```python
from build123d import *

# Parameters (mm, degrees)
SKETCH1_W                                    = 152.4
SKETCH1_H                                    = 88.9
BASE_FLANGE1_DEPTH                           = 1.29032
EDGE_FLANGE1_STRIP_W                         = 5.85978
EDGE_FLANGE1_STRIP_H                         = 1.29032
EDGE_FLANGE1_STRIP_CUT_DEPTH                 = 88.9
EDGE_FLANGE1_STRIP_2_W                       = 5.85978
EDGE_FLANGE1_STRIP_2_H                       = 1.29032
EDGE_FLANGE1_STRIP_CUT_2_DEPTH               = 88.9
EDGE_FLANGE1_DEPTH                           = 88.9
EDGE_FLANGE1_BEND_DEPTH                      = 88.9
F_4_22MM_HOLE_FOR_M3_CLINCH_NUT_D            = 4.22
BREAK_CORNER1_START                          = -77.68082
BREAK_CORNER1_DEPTH                          = 155.36164
CUT_THICKEN1_START                           = 41.91
CUT_THICKEN1_OUTLINE_W                       = 0.127
CUT_THICKEN1_OUTLINE_H                       = 1.29032
CUT_THICKEN1_DEPTH                           = 2.54
CUT_THICKEN2_START                           = 41.91
CUT_THICKEN2_OUTLINE_W                       = 0.127
CUT_THICKEN2_OUTLINE_H                       = 1.29032
CUT_THICKEN2_DEPTH                           = 2.54
MIRROR7_START                                = 41.91
MIRROR7_COPY_1_SKETCH_W                      = 0.127
MIRROR7_COPY_1_SKETCH_H                      = 1.29032
MIRROR7_COPY_1_DEPTH                         = 2.54
MIRROR7_COPY_2_SKETCH_W                      = 0.127
MIRROR7_COPY_2_SKETCH_H                      = 1.29032
MIRROR7_COPY_2_DEPTH                         = 2.54
MOVE_FACE1_BY                                = 1.27
MOVE_FACE1_2_BY                              = 1.27
MOVE_FACE1_3_BY                              = 1.27
MOVE_FACE1_4_BY                              = 1.27
EDGE_FLANGE2_STRIP_W                         = 5.66928
EDGE_FLANGE2_STRIP_H                         = 1.29032
EDGE_FLANGE2_STRIP_CUT_DEPTH                 = 2.54
EDGE_FLANGE2_STRIP_2_W                       = 5.66928
EDGE_FLANGE2_STRIP_2_H                       = 1.29032
EDGE_FLANGE2_STRIP_CUT_2_DEPTH               = 2.54
EDGE_FLANGE2_STRIP_3_W                       = 5.66928
EDGE_FLANGE2_STRIP_3_H                       = 1.29032
EDGE_FLANGE2_STRIP_CUT_3_DEPTH               = 2.54
EDGE_FLANGE2_STRIP_4_W                       = 5.66928
EDGE_FLANGE2_STRIP_4_H                       = 1.29032
EDGE_FLANGE2_STRIP_CUT_4_DEPTH               = 2.54
EDGE_FLANGE2_DEPTH                           = 2.54
EDGE_FLANGE2_BEND_DEPTH                      = 2.54
EDGE_FLANGE2_BEND_2_DEPTH                    = 2.54
EDGE_FLANGE2_BEND_3_DEPTH                    = 2.54
CHANGE_START                                 = -77.68082
CHANGE_NOTE_FOR_REVH_TO_ADD_010_CLEARA_DEPTH = 155.36164


# Read off the part's stored shape, not the designer's step: Break-Corner1, Cut-Thicken1, Cut-Thicken2, change note for revH to add .010" clearance
# Sheet-metal steps are written as plain solids
with BuildPart() as part:
    # Sketch1 → Base-Flange1 (new body)
    with BuildSketch(Plane.XY):
        Rectangle(SKETCH1_W, SKETCH1_H)
    extrude(amount=-BASE_FLANGE1_DEPTH)

    # Edge-Flange1 strip (across the edge) → Edge-Flange1 strip cut (cut)
    with BuildSketch(Plane(origin=(-76.3905, -44.45, -1.29032), x_dir=(1, 0, 0), z_dir=(0, 1, 0))):
        with Locations((-2.67589, -0.64516)):
            Rectangle(EDGE_FLANGE1_STRIP_W, EDGE_FLANGE1_STRIP_H)
    extrude(amount=EDGE_FLANGE1_STRIP_CUT_DEPTH, mode=Mode.SUBTRACT)

    # Edge-Flange1 strip 2 (across the edge) → Edge-Flange1 strip cut 2 (cut)
    with BuildSketch(Plane(origin=(76.3905, 44.45, -1.29032), x_dir=(-1, 0, 0), z_dir=(0, -1, 0))):
        with Locations((-2.67589, -0.64516)):
            Rectangle(EDGE_FLANGE1_STRIP_2_W, EDGE_FLANGE1_STRIP_2_H)
    extrude(amount=EDGE_FLANGE1_STRIP_CUT_2_DEPTH, mode=Mode.SUBTRACT)

    # Edge-Flange1 section (across the edge) → Edge-Flange1 (add)
    with BuildSketch(Plane(origin=(-76.3905, -44.45, -1.29032), x_dir=(1, 0, 0), z_dir=(0, 1, 0))):
        with BuildLine():
            Line((-1.29032, 0.254), (-1.29032, 46.96968))
            Line((-1.29032, 46.96968), (0, 46.96968))
            Line((0, 46.96968), (0, 0.254))
            ThreePointArc((0, 0.254), (0.074394878, 0.074394878), (0.254, 0))
            Line((0.254, 0), (0.254, -1.29032))
            ThreePointArc((0.254, -1.29032), (-0.837999144, -0.837999144), (-1.29032, 0.254))
        make_face()
    extrude(amount=EDGE_FLANGE1_DEPTH)

    # Edge-Flange1 section 2 (across the edge) → Edge-Flange1 bend (add)
    with BuildSketch(Plane(origin=(76.3905, 44.45, -1.29032), x_dir=(-1, 0, 0), z_dir=(0, -1, 0))):
        with BuildLine():
            Line((-1.29032, 0.254), (-1.29032, 46.96968))
            Line((-1.29032, 46.96968), (0, 46.96968))
            Line((0, 46.96968), (0, 0.254))
            ThreePointArc((0, 0.254), (0.074394878, 0.074394878), (0.254, 0))
            Line((0.254, 0), (0.254, -1.29032))
            ThreePointArc((0.254, -1.29032), (-0.837999144, -0.837999144), (-1.29032, 0.254))
        make_face()
    extrude(amount=EDGE_FLANGE1_BEND_DEPTH)

    # Ø4.22mm hole for M3 Clinch nut (through all)
    with Locations(Plane.ZY.offset(77.68082)):
        with Locations((-43.26, 0)):
            f_4_22mm_hole_for_m3_clinch_nut = Hole(F_4_22MM_HOLE_FOR_M3_CLINCH_NUT_D / 2)

    # Mirror1: Ø4.22mm hole for M3 Clinch nut across plane
    add(f_4_22mm_hole_for_m3_clinch_nut.mirror(Plane(origin=(0, 0, 0), x_dir=(0, 0, 1), z_dir=(1, 0, 0))), mode=Mode.SUBTRACT)

    # Break-Corner1 outline → Break-Corner1 (cut)
    with BuildSketch(Plane.YZ.offset(BREAK_CORNER1_START)):
        with BuildLine():
            Line((44.45, -48.26), (44.45, -47.498))
            ThreePointArc((44.45, -47.498), (44.226815367, -48.036815367), (43.688, -48.26))
            Line((43.688, -48.26), (44.45, -48.26))
        make_face()
        with BuildLine():
            Line((-44.45, -48.26), (-43.688, -48.26))
            ThreePointArc((-43.688, -48.26), (-44.226815367, -48.036815367), (-44.45, -47.498))
            Line((-44.45, -47.498), (-44.45, -48.26))
        make_face()
    extrude(amount=BREAK_CORNER1_DEPTH, mode=Mode.SUBTRACT)

    # Cut-Thicken1 outline → Cut-Thicken1 (cut)
    with BuildSketch(Plane(origin=(0, 0, 0), x_dir=(1, 0, 0), z_dir=(0, 1, 0)).offset(CUT_THICKEN1_START)):
        with Locations((36.97732, 0.64516)):
            Rectangle(CUT_THICKEN1_OUTLINE_W, CUT_THICKEN1_OUTLINE_H)
    cut_thicken1 = extrude(amount=CUT_THICKEN1_DEPTH, mode=Mode.SUBTRACT)

    # Cut-Thicken2 outline → Cut-Thicken2 (cut)
    with BuildSketch(Plane(origin=(0, 0, 0), x_dir=(1, 0, 0), z_dir=(0, 1, 0)).offset(CUT_THICKEN2_START)):
        with Locations((39.64432, 0.64516)):
            Rectangle(CUT_THICKEN2_OUTLINE_W, CUT_THICKEN2_OUTLINE_H)
    cut_thicken2 = extrude(amount=CUT_THICKEN2_DEPTH, mode=Mode.SUBTRACT)

    # Mirror6: Cut-Thicken1, Cut-Thicken2 across plane
    add(cut_thicken1.mirror(Plane(origin=(0, 0, 0), x_dir=(0, 0, 1), z_dir=(1, 0, 0))), mode=Mode.SUBTRACT)
    add(cut_thicken2.mirror(Plane(origin=(0, 0, 0), x_dir=(0, 0, 1), z_dir=(1, 0, 0))), mode=Mode.SUBTRACT)

    # Mirror7: Cut-Thicken1, Cut-Thicken2 across plane
    add(cut_thicken1.mirror(Plane.ZX), mode=Mode.SUBTRACT)
    add(cut_thicken2.mirror(Plane.ZX), mode=Mode.SUBTRACT)

    # Mirror7 copy 1 sketch → Mirror7 copy 1 (cut)
    with BuildSketch(Plane(origin=(0, 0, 0), x_dir=(-1, 0, 0), z_dir=(0, -1, 0)).offset(MIRROR7_START)):
        with Locations((36.97732, 0.64516)):
            Rectangle(MIRROR7_COPY_1_SKETCH_W, MIRROR7_COPY_1_SKETCH_H)
    extrude(amount=MIRROR7_COPY_1_DEPTH, mode=Mode.SUBTRACT)

    # Mirror7 copy 2 sketch → Mirror7 copy 2 (cut)
    with BuildSketch(Plane(origin=(0, 0, 0), x_dir=(-1, 0, 0), z_dir=(0, -1, 0)).offset(MIRROR7_START)):
        with Locations((39.64432, 0.64516)):
            Rectangle(MIRROR7_COPY_2_SKETCH_W, MIRROR7_COPY_2_SKETCH_H)
    extrude(amount=MIRROR7_COPY_2_DEPTH, mode=Mode.SUBTRACT)

    # Move Face1: a face moved inward by 1.27
    extrude(part.faces().sort_by_distance((-38.31082, -44.45, -0.64516))[0], amount=MOVE_FACE1_BY, dir=(0, 1, 0), mode=Mode.SUBTRACT)

    # Move Face1 2: a face moved inward by 1.27
    extrude(part.faces().sort_by_distance((38.31082, -44.45, -0.64516))[0], amount=MOVE_FACE1_2_BY, dir=(0, 1, 0), mode=Mode.SUBTRACT)

    # Move Face1 3: a face moved inward by 1.27
    extrude(part.faces().sort_by_distance((-38.31082, 44.45, -0.64516))[0], amount=MOVE_FACE1_3_BY, dir=(0, -1, 0), mode=Mode.SUBTRACT)

    # Move Face1 4: a face moved inward by 1.27
    extrude(part.faces().sort_by_distance((38.31082, 44.45, -0.64516))[0], amount=MOVE_FACE1_4_BY, dir=(0, -1, 0), mode=Mode.SUBTRACT)

    # Edge-Flange2 strip (across the edge) → Edge-Flange2 strip cut (cut)
    with BuildSketch(Plane(origin=(37.04082, 43.18, -1.29032), x_dir=(0, -1, 0), z_dir=(1, 0, 0))):
        with Locations((-1.29032, -0.64516)):
            Rectangle(EDGE_FLANGE2_STRIP_W, EDGE_FLANGE2_STRIP_H)
    extrude(amount=EDGE_FLANGE2_STRIP_CUT_DEPTH, mode=Mode.SUBTRACT)

    # Edge-Flange2 strip 2 (across the edge) → Edge-Flange2 strip cut 2 (cut)
    with BuildSketch(Plane(origin=(-39.58082, 43.18, -1.29032), x_dir=(0, -1, 0), z_dir=(1, 0, 0))):
        with Locations((-1.29032, -0.64516)):
            Rectangle(EDGE_FLANGE2_STRIP_2_W, EDGE_FLANGE2_STRIP_2_H)
    extrude(amount=EDGE_FLANGE2_STRIP_CUT_2_DEPTH, mode=Mode.SUBTRACT)

    # Edge-Flange2 strip 3 (across the edge) → Edge-Flange2 strip cut 3 (cut)
    with BuildSketch(Plane(origin=(39.58082, -43.18, -1.29032), x_dir=(0, 1, 0), z_dir=(-1, 0, 0))):
        with Locations((-1.29032, -0.64516)):
            Rectangle(EDGE_FLANGE2_STRIP_3_W, EDGE_FLANGE2_STRIP_3_H)
    extrude(amount=EDGE_FLANGE2_STRIP_CUT_3_DEPTH, mode=Mode.SUBTRACT)

    # Edge-Flange2 strip 4 (across the edge) → Edge-Flange2 strip cut 4 (cut)
    with BuildSketch(Plane(origin=(-37.04082, -43.18, -1.29032), x_dir=(0, 1, 0), z_dir=(-1, 0, 0))):
        with Locations((-1.29032, -0.64516)):
            Rectangle(EDGE_FLANGE2_STRIP_4_W, EDGE_FLANGE2_STRIP_4_H)
    extrude(amount=EDGE_FLANGE2_STRIP_CUT_4_DEPTH, mode=Mode.SUBTRACT)

    # Edge-Flange2 section (across the edge) → Edge-Flange2 (add)
    with BuildSketch(Plane(origin=(37.04082, 43.18, -1.29032), x_dir=(0, -1, 0), z_dir=(1, 0, 0))):
        with BuildLine():
            Line((0, 0.254), (0, 1.27))
            Line((0, 1.27), (1.29032, 1.27))
            Line((1.29032, 1.27), (1.29032, 0.254))
            ThreePointArc((1.29032, 0.254), (1.364714878, 0.074394878), (1.54432, 0))
            Line((1.54432, 0), (1.54432, -1.29032))
            ThreePointArc((1.54432, -1.29032), (0.452320856, -0.837999144), (0, 0.254))
        make_face()
    extrude(amount=EDGE_FLANGE2_DEPTH)

    # Edge-Flange2 section 2 (across the edge) → Edge-Flange2 bend (add)
    with BuildSketch(Plane(origin=(-39.58082, 43.18, -1.29032), x_dir=(0, -1, 0), z_dir=(1, 0, 0))):
        with BuildLine():
            Line((0, 0.254), (0, 1.27))
            Line((0, 1.27), (1.29032, 1.27))
            Line((1.29032, 1.27), (1.29032, 0.254))
            ThreePointArc((1.29032, 0.254), (1.364714878, 0.074394878), (1.54432, 0))
            Line((1.54432, 0), (1.54432, -1.29032))
            ThreePointArc((1.54432, -1.29032), (0.452320856, -0.837999144), (0, 0.254))
        make_face()
    extrude(amount=EDGE_FLANGE2_BEND_DEPTH)

    # Edge-Flange2 section 3 (across the edge) → Edge-Flange2 bend 2 (add)
    with BuildSketch(Plane(origin=(39.58082, -43.18, -1.29032), x_dir=(0, 1, 0), z_dir=(-1, 0, 0))):
        with BuildLine():
            Line((0, 0.254), (0, 1.27))
            Line((0, 1.27), (1.29032, 1.27))
            Line((1.29032, 1.27), (1.29032, 0.254))
            ThreePointArc((1.29032, 0.254), (1.364714878, 0.074394878), (1.54432, 0))
            Line((1.54432, 0), (1.54432, -1.29032))
            ThreePointArc((1.54432, -1.29032), (0.452320856, -0.837999144), (0, 0.254))
        make_face()
    extrude(amount=EDGE_FLANGE2_BEND_2_DEPTH)

    # Edge-Flange2 section 4 (across the edge) → Edge-Flange2 bend 3 (add)
    with BuildSketch(Plane(origin=(-37.04082, -43.18, -1.29032), x_dir=(0, 1, 0), z_dir=(-1, 0, 0))):
        with BuildLine():
            Line((0, 0.254), (0, 1.27))
            Line((0, 1.27), (1.29032, 1.27))
            Line((1.29032, 1.27), (1.29032, 0.254))
            ThreePointArc((1.29032, 0.254), (1.364714878, 0.074394878), (1.54432, 0))
            Line((1.54432, 0), (1.54432, -1.29032))
            ThreePointArc((1.54432, -1.29032), (0.452320856, -0.837999144), (0, 0.254))
        make_face()
    extrude(amount=EDGE_FLANGE2_BEND_3_DEPTH)

    # change note for revH to add .010_ cl 2 → change note for revH to add .010" clearance (cut)
    with BuildSketch(Plane.YZ.offset(CHANGE_START)):
        with BuildLine():
            Line((43.688, -48.006), (-43.688, -48.006))
            ThreePointArc((-43.688, -48.006), (-44.226815367, -47.782815367), (-44.45, -47.244))
            Line((-44.45, -47.244), (-44.45, -47.498))
            ThreePointArc((-44.45, -47.498), (-44.226815367, -48.036815367), (-43.688, -48.26))
            Line((-43.688, -48.26), (43.688, -48.26))
            ThreePointArc((43.688, -48.26), (44.226815367, -48.036815367), (44.45, -47.498))
            Line((44.45, -47.498), (44.45, -47.244))
            ThreePointArc((44.45, -47.244), (44.226815367, -47.782815367), (43.688, -48.006))
        make_face()
    extrude(amount=CHANGE_NOTE_FOR_REVH_TO_ADD_010_CLEARA_DEPTH, mode=Mode.SUBTRACT)


solid = part.part
```
Could you check a few things on this model? Use its own coordinates, in mm. A direction names the side the tool comes from. Give positions to 0.01 mm unless a question says otherwise; leave off trailing zeros. Loops run counter-clockwise (first coordinate to the right, second up) from the corner with the lowest first, then second, coordinate; pieces in that order, holes last. Notation, with made-up numbers: (-39.5, 18.5) -> (-28.5, 18.5) arc R21 cw to (-28.5, 36.5) -> close; hole circle Ø10 at (-5.5, -40). An arc over 180 degrees is marked (long way). Put each result on its own line as item: value.
(1) For faces 4 (the face through (-76.39, -1, -25)), 5 (the face through (-77, -44.45, -13)), which set-ups out of +Z, -Z, +X, -X, +Y, -Y let a thin tool reach every point of the face, with its end or its side?
Computed:
face 4: -Z, +Y, -Y
face 5: +Z, -Z, +X, -X, -Y
(2) Imagine slicing it at A-A on y = 0. Write out the boundary of the cut face in (x, z), plus the area to 3 significant figures.
Computed:
outline: (-77.68, -48.01) -> (-76.39, -48.01) -> (-76.39, -45.37) -> (-77.68, -45.37) -> close; (-77.68, -41.15) -> (-76.39, -41.15) -> (-76.39, -1.54) arc R0.25 cw to (-76.14, -1.29) -> (76.14, -1.29) arc R0.25 cw to (76.39, -1.54) -> (76.39, -41.15) -> (77.68, -41.15) -> (77.68, -1.54) arc R1.54 ccw to (76.14, 0) -> (-76.14, 0) arc R1.54 ccw to (-77.68, -1.54) -> close; (76.39, -48.01) -> (77.68, -48.01) -> (77.68, -45.37) -> (76.39, -45.37) -> close
area: 309 mm^2
(3) Imagine slicing it at D-D on y = -18.5. Write out the boundary of the cut face in (x, z).
Computed:
outline: (-77.68, -48.01) -> (-76.39, -48.01) -> (-76.39, -1.54) arc R0.25 cw to (-76.14, -1.29) -> (76.14, -1.29) arc R0.25 cw to (76.39, -1.54) -> (76.39, -48.01) -> (77.68, -48.01) -> (77.68, -1.54) arc R1.54 ccw to (76.14, 0) -> (-76.14, 0) arc R1.54 ccw to (-77.68, -1.54) -> close
(4) Thinking about a two-plate mould opening in Y: for faces 1 (the face through (77.04, 0.09, -41.15)), 2 (the face through (76.39, 1, -25)), 3 (the face through (77, -44.45, -13)), which applies, pulls with the +Y half, pulls with the -Y half, needs draft (parallel to the pull), parting line crosses it, or undercut?
Computed:
face 1: undercut
face 2: needs draft
face 3: pulls with the -Y half
(5) Please list where these lines run through material, in increasing order: probe 1 along X at (y, z) = (-22, -35); probe 2 along Y at (x, z) = (76.7, -43.26); probe 3 along Z at (x, y) = (-42, -17). Write a range as [from, to].
Computed:
probe 1: [-77.68, -76.39], [76.39, 77.68]
probe 2: [-44.45, -2.11], [2.11, 44.45]
probe 3: [-1.29, 0]
(6) Imagine slicing it at C-C on z = -7. Write out the boundary of the cut face in (x, y), plus the area to 3 significant figures.
Computed:
outline: (-77.68, -44.45) -> (-76.39, -44.45) -> (-76.39, 44.45) -> (-77.68, 44.45) -> close; (76.39, -44.45) -> (77.68, -44.45) -> (77.68, 44.45) -> (76.39, 44.45) -> close
area: 229 mm^2
(7) Imagine slicing it at B-B on z = -43.26. Write out the boundary of the cut face in (x, y).
Computed:
outline: (-77.68, -44.45) -> (-76.39, -44.45) -> (-76.39, -2.11) -> (-77.68, -2.11) -> close; (-77.68, 2.11) -> (-76.39, 2.11) -> (-76.39, 44.45) -> (-77.68, 44.45) -> close; (76.39, -44.45) -> (77.68, -44.45) -> (77.68, -2.11) -> (76.39, -2.11) -> close; (76.39, 2.11) -> (77.68, 2.11) -> (77.68, 44.45) -> (76.39, 44.45) -> close
(8) I'm going to push a flat-ended pin straight in: pin 1 Ø1 at (x, y) = (38.5, 42.5) entering from -Z. Where does the tip first touch, or does it pass through?
Computed:
pin 1: z = -2.56
